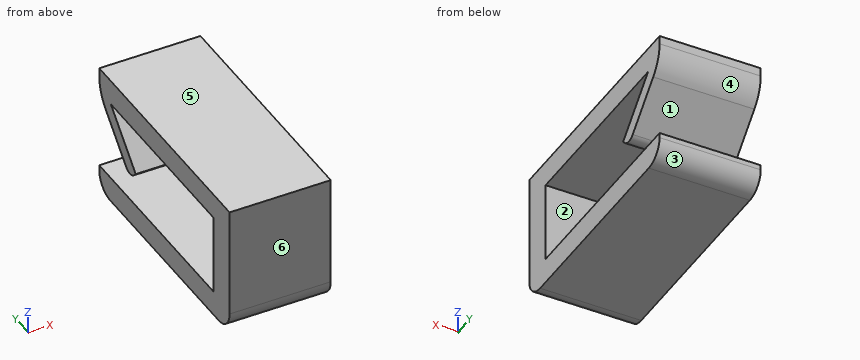
Autodesk Inventor part; units mm, degrees
ref_plane "YZ Plane" through (0, 0, 0) normal (1, 0, 0) x (0, 1, 0)
ref_plane "XZ Plane" through (0, 0, 0) normal (0, 1, 0) x (-1, 0, 0)
ref_plane "XY Plane" through (0, 0, 0) normal (0, 0, 1) x (1, 0, 0)
ref_plane "Work Plane1" through (150, 0, -50) normal (0, 0, -1) x (-1, 0, 0)
sketch "Sketch1" plane through (150, 0, -50) normal (0, 0, -1) x (-1, 0, 0)
  line L0 (-107, 15) -> (222, 15)
  line L1 (44.694, 5) -> (34.694, 5)
  line L2 (34.694, 5) -> (34.694, 25)
  line L3 (34.694, 25) -> (44.694, 25)
  line L4 (44.694, 25) -> (44.694, 5)
  line L5 (44.694, 5) -> (34.694, 25) construction
  line L6 (34.694, 5) -> (44.694, 25) construction
  line L7 (34.694, 5) -> (44.694, 5)
  line L8 (44.694, 5) -> (44.694, 1)
  line L9 (44.694, 1) -> (34.694, 1)
  line L10 (34.694, 1) -> (34.694, 5)
  point P0 (150, 0)
  point P1 (39.694, 15)
  dimension "d0" = 20
  dimension "d1" = 10
  dimension "d2" = 177.306
  dimension "d3" = 4
extrude "Extrusion1" add sketch "Sketch1" along normal blind 2.5
sketch "Sketch2" plane through (150, 0, -52.5) normal (0, 0, -1) x (-1, 0, 0)
  line L0 (34.694, 25) -> (34.694, 1)
  line L1 (34.694, 1) -> (44.694, 1)
  line L2 (44.694, 1) -> (44.694, 25)
  line L3 (44.694, 25) -> (34.694, 25)
  line L4 (34.694, 1) -> (44.694, 1)
  line L5 (44.694, 1) -> (44.694, 4)
  line L6 (44.694, 4) -> (34.694, 4)
  line L7 (34.694, 4) -> (34.694, 1)
  point P0 (150, 0)
  dimension "d6" = 3
extrude "Extrusion2" add sketch "Sketch2" along normal blind 8 contours L6 L2 L1 L0
sketch "Sketch3" plane through (150, 0, -60.5) normal (0, 0, -1) x (-1, 0, 0)
  line L0 (34.694, 4) -> (34.694, 1)
  line L1 (34.694, 1) -> (44.694, 1)
  line L2 (44.694, 1) -> (44.694, 4)
  line L3 (44.694, 4) -> (34.694, 4)
  line L4 (-107, 15) -> (222, 15)
  line L5 (34.694, 4) -> (44.694, 4)
  line L6 (44.694, 4) -> (44.694, 25)
  line L7 (44.694, 25) -> (34.694, 25)
  line L8 (34.694, 25) -> (34.694, 4)
  line L9 (34.694, 25) -> (44.694, 25)
  line L10 (44.694, 25) -> (44.694, 1)
  line L11 (44.694, 1) -> (34.694, 1)
  line L12 (34.694, 1) -> (34.694, 25)
  point P0 (150, 0)
extrude "Extrusion3" add sketch "Sketch3" along normal blind 2.5
sketch "Sketch4" plane through (115.306, 1, -50) normal (1, 0, 0) x (0, 0, -1)
  line L0 (2.5, 3) -> (2.5, 24)
  line L1 (2.5, 24) -> (8.1569, 18.3431)
  line L2 (2.5, 24) -> (10.5, 24) construction
  line L3 (8.1569, 18.3431) -> (7.0962, 17.2825)
  line L4 (7.0962, 17.2825) -> (2.5, 21.8787)
  point P0 (-50, -1)
  dimension "d11" = 8
  dimension "d12" = 45
  dimension "d13" = 1.5
extrude "Extrusion4" add sketch "Sketch4" against normal up to surface (10 mm away)
fillet "Fillet1" radius 2 2 edges at (110.306, 25, -63) (110.306, 1, -63)
fillet "Fillet2" radius 4 1 edges at (110.306, 25, -52.5)
fillet "Fillet3" radius 1 1 edges at (110.306, 19.3431, -58.1569)
properties part number "cable-clip_3DPrint"
CAD build for the part. Positions are in the model's coordinates, mm. Face numbers are marked on the shaded views. A direction names the side the tool comes from. Coordinates: 2 decimals unless noted, no trailing zeros. Order: outer loops, then holes, each group sorted by start corner. A loop starts at its lowest first (then second) coordinate and runs counter-clockwise, first axis right, second up.
(1) Drill centre lines: L1, parallel to Z at x = 109.25, y = 15.5; L2, parallel to Z at x = 106.25, y = 19.5; L3, parallel to Z at x = 110.25, y = 21. Where is each one in solid material? Low to high.
Solution:
L1: z = -63 to -60.5, -52.5 to -50
L2: z = -63 to -60.5, -57.73 to -55.88, -52.5 to -50
L3: z = -63 to -60.5, -56.5 to -54.38, -52.5 to -50
(2) Mould opens along Z. For the marked faces 4, 5 and 6 say: released by +Z, released by -Z, zero draft, split by the parting line, or undercut.
Solution:
face 4: undercut
face 5: released by +Z
face 6: zero draft
(3) Saw through at B-B, the plane z = -56.5. Write the cut outline in (x, y), and give its area (3 significant figures).
Solution:
outline: (105.31, 1) - (115.31, 1) - (115.31, 4) - (105.31, 4) - close; (105.31, 18.88) - (115.31, 18.88) - (115.31, 21) - (105.31, 21) - close
area: 51.2 mm2
(4) Saw through at D-D, the plane y = 19.25. Write the cut outline in (x, z).
Solution:
outline: (105.31, -63) - (115.31, -63) - (115.31, -60.5) - (105.31, -60.5) - close; (105.31, -57.74) - (115.31, -57.74) - (115.31, -56.13) - (105.31, -56.13) - close; (105.31, -52.5) - (115.31, -52.5) - (115.31, -50) - (105.31, -50) - close
(5) Saw through at A-A, the plane y = 7.25. Write the cut outline in (x, z).
Solution:
outline: (105.31, -63) - (115.31, -63) - (115.31, -60.5) - (105.31, -60.5) - close; (105.31, -52.5) - (115.31, -52.5) - (115.31, -50) - (105.31, -50) - close
(6) Saw through at C-C, the plane x = 107.25. Write the cut outline in (y, z), and give its area (3 significant figures).
Solution:
outline: (1, -61) arc R2 ccw to (3, -63) - (23, -63) arc R2 ccw to (25, -61) - (25, -60.5) - (4, -60.5) - (4, -52.5) - (22.88, -52.5) - (18.28, -57.1) - (18.64, -57.45) arc R1 ccw to (20.05, -57.45) - (23.83, -53.67) arc R4 ccw to (25, -50.84) - (25, -50) - (1, -50) - close
area: 153 mm2
(7) Which spindle directions (+Z, -Z, +X, -X, +Y, -Y) get a long thin tool onto all of the face, cutting with end or side? Do the marked faces 1, 2 and 3. Say none if no direction does.
Solution:
face 1: +X, -X, +Y
face 2: +X, -X
face 3: -Z, +X, -X, +Y
